from build123d import *

# Parameters (mm, degrees)
ESBO_O1_R                = 5
RESSALTO_EXTRUS_O1_DEPTH = 4
ESBO_O4_R                = 2.5
RESSALTO_EXTRUS_O2_DEPTH = 6.5
ESBO_O5_R                = 3
RESSALTO_EXTRUS_O4_DEPTH = 1.5


with BuildPart() as part:
    # Esboço1 → Ressalto-extrusão1 (new body)
    with BuildSketch(Plane(origin=(0, 0, 0), x_dir=(1, 0, 0), z_dir=(0, 1, 0))):
        with Locations(Location((0, 0, 0), (0, 0, 270))):
            Circle(ESBO_O1_R)
    extrude(amount=RESSALTO_EXTRUS_O1_DEPTH)

    # Esboço4 → Ressalto-extrusão2 (add)
    with BuildSketch(Plane(origin=(0, 0, 0), x_dir=(-1, 0, 0), z_dir=(0, -1, 0))):
        with Locations(Location((0, 0, 0), (0, 0, 270))):
            Circle(ESBO_O4_R)
    extrude(amount=RESSALTO_EXTRUS_O2_DEPTH)

    # Esboço5 → Ressalto-extrusão4 (add)
    with BuildSketch(Plane.XZ):
        with Locations(Location((0, 0, 0), (0, 0, 90))):
            Circle(ESBO_O5_R)
    extrude(amount=RESSALTO_EXTRUS_O4_DEPTH)

    # Esboço7 → Broca de rosquear para tarraxa de M31 (revolve, cut)
    with BuildSketch(Plane(origin=(0, -6.5, 0), x_dir=(0, 0, -1), z_dir=(1, 0, 0))):
        Polygon((0, 0), (0, 8.751075774), (1.25, 8), (1.25, 0), align=None)
    revolve(axis=Axis((0, -12.85, 0), (0, 1, 0)), mode=Mode.SUBTRACT)


solid = part.part
Model file for the job. Use its own axes, mm. A direction names the side the tool comes from. Give positions to 0.01 mm unless a question says otherwise; leave off trailing zeros. Loops run counter-clockwise (first coordinate to the right, second up) from the corner with the lowest first, then second, coordinate; pieces in that order, holes last.
1) Saw through at B-B (y = 1.25). Write the cut outline in (x, z), plus the area to 3 significant figures.
2) Tool access for faces 4 (the flat face through (0, 4, 0)), 5 (the cylindrical face through (-0.9, -0.74, 2.86)): list every direction of +Z, -Z, +X, -X, +Y, -Y with a clear straight run to the whole face (end or side of a thin tool).
3) Pull direction Z, two halves, no side cores. Call faces 1 (the flat face through (-1, -6.5, 1)), 2 (the cylindrical face through (1.22, -2.56, 0.27)), 3 (the cylindrical face through (-4.88, 1.97, -1.08)): +Z half, -Z half, draft (parallel to the pull), parting line (faces both ways), or undercut.
4) Flat gauge pins, fed straight in: pin 1 Ø1.8 at (x, z) = (0, 0) entering from -Y; pin 2 Ø1.5 at (x, z) = (-2, -3) entering from -Y; pin 3 Ø6 at (x, y) = (-1.5, 0) entering from +Z; pin 4 Ø5 at (x, y) = (3, -3) entering from +Z. Where does each tip first touch, or does it go through?
5) Saw through at C-C (z = 2.75). Write the cut outline in (x, y).
6) Saw through at D-D (y = 2.5). Write the cut outline in (x, z).
7) Wall check: line 1 (X direction, y = -0.25, z = 0); line 2 (X direction, y = -4, z = 0); line 3 (Y direction, x = 4, z = 0.75). Give the ranges that are in metal, low to high.
8) Saw through at A-A (x = 1.5). Write the cut outline in (y, z), plus the area to 3 significant figures.
Answer block:
1. outline: circle Ø10 at (0, 0); hole circle Ø2.5 at (0, 0)
1. area: 73.6 mm2
2. face 4: +Z, -Z, +X, -X, +Y
2. face 5: -Y
3. face 1: draft
3. face 2: undercut
3. face 3: parting line
4. pin 1: stops at y = 1.71
4. pin 2: stops at y = -1.5
4. pin 3: stops at z = 5
4. pin 4: stops at z = 2.83
5. outline: (-4.18, 0) - (-1.2, 0) - (-1.2, -1.5) - (1.2, -1.5) - (1.2, 0) - (4.18, 0) - (4.18, 4) - (-4.18, 4) - close
6. outline: circle Ø10 at (0, 0)
7. line 1: x = -3 to -1.25, 1.25 to 3
7. line 2: x = -2.5 to -1.25, 1.25 to 2.5
7. line 3: y = 0 to 4
8. outline: (-6.5, -2) - (-1.5, -2) - (-1.5, -2.6) - (0, -2.6) - (0, -4.77) - (4, -4.77) - (4, 4.77) - (0, 4.77) - (0, 2.6) - (-1.5, 2.6) - (-1.5, 2) - (-6.5, 2) - close
8. area: 66.0 mm2
